from build123d import *

# Parameters (mm, degrees)
BOSS_EXTRUDE1_DEPTH = 76.2
SKETCH2_W           = 6.985
SKETCH2_H           = 9.525
CUT_EXTRUDE1_DEPTH  = 119.84173867
CUT_EXTRUDE2_DEPTH  = 119.84173867
CUT_EXTRUDE3_DEPTH  = 119.84173867
FILLET1_R           = 2.54
CUT_EXTRUDE4_DEPTH  = 5.08
CUT_EXTRUDE6_DEPTH  = 15.113
FILLET2_R           = 0.508
BOSS_EXTRUDE2_DEPTH = 15.5575
BOSS_EXTRUDE3_DEPTH = 5.08
CUT_EXTRUDE7_DEPTH  = 5.08


with BuildPart() as part:
    # Sketch1 → Boss-Extrude1 (new body)
    with BuildSketch(Plane.XY):
        Polygon((-15.5575, 76.2), (15.5575, 76.2), (15.5575, -76.2), (7.845485509, -76.2), (9.525, -85.725), (-9.525, -85.725), (-7.845485509, -76.2), (-15.5575, -76.2), align=None)
    extrude(amount=BOSS_EXTRUDE1_DEPTH)

    # Sketch2 → Cut-Extrude1 (cut, through all)
    with BuildSketch(Plane(origin=(15.5575, 0, 0), x_dir=(0, 0, -1), z_dir=(1, 0, 0))):
        with Locations((-3.4925, -80.9625)):
            Rectangle(SKETCH2_W, SKETCH2_H)
    extrude(amount=-CUT_EXTRUDE1_DEPTH, mode=Mode.SUBTRACT)

    # Sketch3 → Cut-Extrude2 (cut, through all)
    with BuildSketch(Plane(origin=(15.5575, 0, 0), x_dir=(0, 0, -1), z_dir=(1, 0, 0))):
        with BuildLine():
            Line((-76.2, -85.725), (-76.2, -76.2))
            Line((-76.2, -76.2), (-76.2, 76.2))
            Line((-76.2, 76.2), (-6.541803462, 76.2))
            ThreePointArc((-6.541803462, 76.2), (-58.046669251, 2.411215556), (-76.2, -85.725))
        make_face()
        with BuildLine():
            Line((0, -76.2), (0, 67.75939176))
            ThreePointArc((0, 67.75939176), (-18.20597202, -4.22030412), (0, -76.2))
        make_face()
    extrude(amount=-CUT_EXTRUDE2_DEPTH, mode=Mode.SUBTRACT)

    # Sketch6 → Cut-Extrude3 (cut, through all)
    with BuildSketch(Plane(origin=(15.5575, 0, 0), x_dir=(0, 0, -1), z_dir=(1, 0, 0))):
        with BuildLine():
            ThreePointArc((-28.934409948, -61.883434575), (-23.879909813, -60.517759582), (-22.716254779, -55.412963136))
            ThreePointArc((-22.716254779, -55.412963136), (-30.753414225, -11.294498854), (-26.546552055, 33.352305435))
            ThreePointArc((-26.546552055, 33.352305435), (-49.181053892, -9.446405872), (-61.429710833, -56.286781256))
            ThreePointArc((-61.429710833, -56.286781256), (-59.737369376, -60.827463042), (-55.008021131, -61.883434575))
            ThreePointArc((-55.008021131, -61.883434575), (-41.971215539, -60.062859411), (-28.934409948, -61.883434575))
        make_face()
    extrude(amount=-CUT_EXTRUDE3_DEPTH, mode=Mode.SUBTRACT)

    # Fillet1
    fillet1_edges = [part.edges().sort_by_distance(p)[0] for p in [
        (0, 33.352305435, 26.546552055),
    ]]
    fillet(fillet1_edges, radius=FILLET1_R)

    # Sketch7 → Cut-Extrude4 (cut, symmetric)
    with BuildSketch(Plane(origin=(0, 0, 0), x_dir=(0, 0, -1), z_dir=(1, 0, 0))):
        with BuildLine():
            Line((-30.699128799, 4.016230293), (-17.981752538, 4.016230293))
            ThreePointArc((-17.981752538, 4.016230293), (-17.415803594, -19.667907964), (-13.161921654, -42.973769707))
            Line((-13.161921654, -42.973769707), (-26.264177108, -42.973769707))
            ThreePointArc((-26.264177108, -42.973769707), (-30.179968378, -19.639057999), (-30.699128799, 4.016230293))
        make_face()
    extrude(amount=CUT_EXTRUDE4_DEPTH, both=True, mode=Mode.SUBTRACT)

    # Sketch10 → Cut-Extrude6 (cut, symmetric)
    with BuildSketch(Plane(origin=(15.5575, 76.2, 6.541803462), x_dir=(-1, 0, 0), z_dir=(0, -0.7903999954772005, -0.6125910929401777))):
        Polygon((0, 5.170641427), (6.985, 5.170641427), (0, -3.655858573), align=None)
        Polygon((31.115, 5.170641427), (31.115, -3.655858573), (24.13, 5.170641427), align=None)
    extrude(amount=CUT_EXTRUDE6_DEPTH, both=True, mode=Mode.SUBTRACT)

    # Fillet2
    fillet2_edges = [part.edges().sort_by_distance(p)[0] for p in [
        (0, 76.2, 6.541803462),
        (-14.111333502, 74.930435776, 7.871138317),
        (14.111333502, 74.930435776, 7.871138317),
        (-15.5575, 5.090891194, 56.873019023),
        (15.5575, 5.090891194, 56.873019023),
    ]]
    fillet(fillet2_edges, radius=FILLET2_R)


with BuildPart() as body_2:
    # Sketch11 → Boss-Extrude2 (new body)
    with BuildSketch(Plane(origin=(15.5575, 0, 0), x_dir=(0, 0, -1), z_dir=(1, 0, 0))):
        with BuildLine():
            ThreePointArc((-61.429710833, -56.286781256), (-59.737369376, -60.827463042), (-55.008021131, -61.883434575))
            ThreePointArc((-55.008021131, -61.883434575), (-41.971215539, -60.062859411), (-28.934409948, -61.883434575))
            ThreePointArc((-28.934409948, -61.883434575), (-23.879909813, -60.517759582), (-22.716254779, -55.412963136))
            ThreePointArc((-22.716254779, -55.412963136), (-30.33926448, -17.846197276), (-29.038721333, 20.464124591))
            ThreePointArc((-29.038721333, 20.464124591), (-30.691356883, 23.236746406), (-33.730314595, 22.14891737))
            ThreePointArc((-33.730314595, 22.14891737), (-51.496194807, -15.685940761), (-61.429710833, -56.286781256))
        make_face()
        with BuildLine():
            ThreePointArc((-57.657212561, -56.820032407), (-57.234127197, -57.955202853), (-56.051790136, -58.219195736))
            ThreePointArc((-56.051790136, -58.219195736), (-41.971215539, -56.252859411), (-27.890640943, -58.219195736))
            ThreePointArc((-27.890640943, -58.219195736), (-26.62701591, -57.877776988), (-26.336102151, -56.601577877))
            ThreePointArc((-26.336102151, -56.601577877), (-33.838316864, -21.365349504), (-33.651053161, 14.660196264))
            ThreePointArc((-33.651053161, 14.660196264), (-48.944068981, -19.975014906), (-57.657212561, -56.820032407))
        make_face(mode=Mode.SUBTRACT)
    extrude(amount=-BOSS_EXTRUDE2_DEPTH)

    # Sketch13 → Cut-Extrude7 (cut, symmetric)
    with BuildSketch(Plane(origin=(0, 0, 0), x_dir=(0, 0, -1), z_dir=(1, 0, 0))):
        with BuildLine():
            Line((-17.981752538, 4.016230293), (-34.513828125, 4.016230293))
            ThreePointArc((-34.513828125, 4.016230293), (-34.007192205, -19.631694302), (-30.182465628, -42.973769707))
            Line((-30.182465628, -42.973769707), (-13.161921654, -42.973769707))
            ThreePointArc((-13.161921654, -42.973769707), (-17.415803594, -19.667907964), (-17.981752538, 4.016230293))
        make_face()
    extrude(amount=CUT_EXTRUDE7_DEPTH, both=True, mode=Mode.SUBTRACT)


with BuildPart() as body_3:
    # Sketch12 → Boss-Extrude3 (new body)
    with BuildSketch(Plane(origin=(15.5575, 0, 0), x_dir=(0, 0, -1), z_dir=(1, 0, 0))):
        with BuildLine():
            ThreePointArc((-23.831738773, 27.962776346), (-26.492538641, 32.964962799), (-31.905127941, 31.28996957))
            ThreePointArc((-31.905127941, 31.28996957), (-53.570754409, -11.710044351), (-65.056281593, -58.469890723))
            ThreePointArc((-65.056281593, -58.469890723), (-62.925669808, -64.071096093), (-57.083298558, -65.405152448))
            ThreePointArc((-57.083298558, -65.405152448), (-41.422387692, -63.30256815), (-25.761476826, -65.405152448))
            ThreePointArc((-25.761476826, -65.405152448), (-19.442461008, -63.610654229), (-18.093267187, -57.18182379))
            ThreePointArc((-18.093267187, -57.18182379), (-26.733177439, -14.998448579), (-23.831738773, 27.962776346))
        make_face()
        with BuildLine():
            ThreePointArc((-27.890640943, -58.219195736), (-26.62701591, -57.877776988), (-26.336102151, -56.601577877))
            ThreePointArc((-26.336102151, -56.601577877), (-33.838316864, -21.365349504), (-33.651053161, 14.660196264))
            ThreePointArc((-33.651053161, 14.660196264), (-48.944068981, -19.975014906), (-57.657212561, -56.820032407))
            ThreePointArc((-57.657212561, -56.820032407), (-57.234127197, -57.955202853), (-56.051790136, -58.219195736))
            ThreePointArc((-56.051790136, -58.219195736), (-41.971215539, -56.252859411), (-27.890640943, -58.219195736))
        make_face(mode=Mode.SUBTRACT)
    extrude(amount=BOSS_EXTRUDE3_DEPTH)


with BuildPart() as body_2_1:
    add(body_2.part)

    # Combine1: union body 3
    add(body_3.part)


with BuildPart() as body_2_2:
    # Mirror1: mirrored copy
    add(body_2_1.part.mirror(Plane(origin=(0, -71.361391395, -45.215986197), x_dir=(0, 0, 1), z_dir=(1, 0, 0))))


solid = body_2_2.part
Geometry: final body of the model. Coordinates: model frame, mm. A direction names the side the tool comes from. Round coordinates to 2 decimals unless told otherwise and drop trailing zeros. Loops run counter-clockwise (first coordinate to the right, second up) from the corner with the lowest first, then second, coordinate; pieces in that order, holes last. Notation, with made-up numbers: M -17,39.5 L 23,39.5 A21 ccw 23,53.5 Z; hole C -11.75,-5 d2. An arc over 180 degrees is marked long. One line per question, with ' | ' between items.
(1) Contact query for flat-ended pins moving along their axis: P1, Ø6, axis at x = -17, z = 50, coming from the -Y side; P2, Ø6, axis at y = 12.5, z = 38.5, coming from the +X side; P3, Ø14, axis at y = -26, z = 42.5, coming from the +X side; P4, Ø1.1, axis at x = -2, z = 32, coming from the -Y side. Output: stop coordinate, or through.
Check result:
P1: stops at y = -64.44 | P2: stops at x = 0 | P3: passes through | P4: stops at y = -61.24
(2) Cut plane A-A on z = 36. Return the cut outline in (x, y), plus the area to 3 significant figures.
Check result:
outline: M -20.64,-63.55 L -15.56,-63.55 L -15.56,-60.44 L 0,-60.44 L 0,-56.6 L -20.64,-56.6 Z; M -20.64,10.32 L 0,10.32 L 0,18.26 L -15.56,18.26 L -15.56,24.78 L -20.64,24.78 Z | area: 292 mm2
(3) Cut plane B-B on y = -16.5. Return the cut outline in (x, z).
Check result:
outline: M -20.64,26.62 L -15.56,26.62 L -15.56,30.45 L -5.08,30.45 L -5.08,34.27 L -20.64,34.27 Z; M -20.64,47.74 L 0,47.74 L 0,51.78 L -15.56,51.78 L -15.56,55.28 L -20.64,55.28 Z
(4) Cut plane C-C on x = -14.25. Return the cut outline in (y, z) (3 decimals).
Check result:
outline: M -61.883,28.934 A5.08 ccw -55.413,22.716 A164.094 cw 20.464,29.039 A2.54 ccw 22.149,33.73 A210.332 ccw -56.287,61.43 A5.08 ccw -61.883,55.008 A47.587 cw Z; hole M -58.219,27.891 A1.27 ccw -56.602,26.336 A167.904 cw 14.66,33.651 A206.522 ccw -56.82,57.657 A1.27 ccw -58.219,56.052 A51.397 cw Z
(5) Material intervals for line 1 along X through (y, z) = (15, 39.5); line 2 along Z through (x, y) = (-15.25, -38.5); line 3 along Z through (x, y) = (-15.25, -14), sorted ascending. Write a range as from..to.
Check result:
line 1: x = -20.64..-15.56 | line 2: z = 27.29..31.18, 54.22..58.13 | line 3: z = 30.61..34.43, 46.83..50.89
(6) Cut plane D-D on y = 18.5. Return the cut outline in (x, z).
Check result:
outline: M -20.64,25.48 L -15.56,25.48 L -15.56,29.33 L 0,29.33 L 0,35.86 L -15.56,35.86 L -15.56,39.65 L -20.64,39.65 Z
(7) Access query for faces 5 (the cylindrical face through (-7.888, -60.063, 42.156)), 6 (the cylindrical face through (-7.89, -15.13, 51.3)), 7 (the flat face through (-3, -42.974, 28)). Directions: +Z, -Z, +X, -X, +Y, -Y. A direction counts if a zero-diameter tool reaches every point of the face in a straight line with its end or side. Return the directions, or none.
Check result:
face 5: +X, -Y | face 6: +Z, +X, +Y | face 7: -Z, +X
(8) Pull-direction query (Y, two-part tool) for faces 1 (the cylindrical face through (-7.89, -60.57, 23.93)), 2 (the flat face through (-5.08, -19, 31)), 3 (the cylindrical face through (-18.062, -11.077, 53.336)), 4 (the cylindrical face through (-10.174, -56.253, 42.171)); classes: +Y half, -Y half, draft (parallel to the pull), parting line (faces both ways), or undercut.
Check result:
face 1: parting line | face 2: undercut | face 3: +Y half | face 4: undercut
